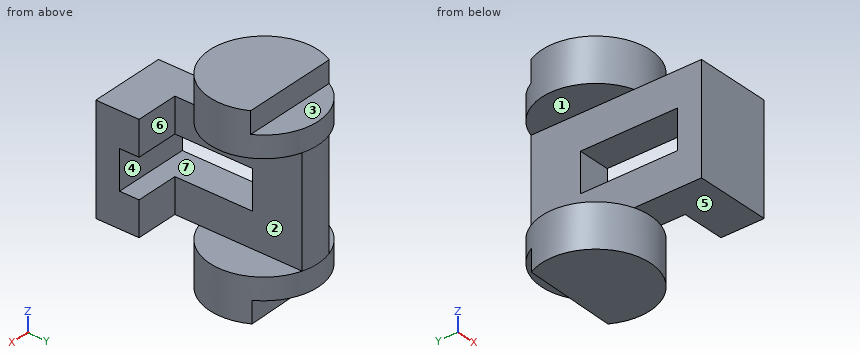
from build123d import *

# Parameters (mm, degrees)
BOSS_EXTRUDE1_DEPTH = 20
BOSS_EXTRUDE2_DEPTH = 50
SKETCH3_W           = 18
SKETCH3_H           = 45
CUT_EXTRUDE1_DEPTH  = 50
SKETCH4_R           = 25
BOSS_EXTRUDE3_DEPTH = 20
CUT_EXTRUDE2_START  = -10
CUT_EXTRUDE2_DEPTH  = 10
BOSS_EXTRUDE4_START = 50
BOSS_EXTRUDE4_DEPTH = 50
BOSS_EXTRUDE5_START = 20
SKETCH7_R           = 25
BOSS_EXTRUDE5_DEPTH = 20
CUT_EXTRUDE3_DEPTH  = 10


with BuildPart() as part:
    # Sketch1 → Boss-Extrude1 (new body)
    with BuildSketch(Plane(origin=(0, 0, 0), x_dir=(0, 0, -1), z_dir=(1, 0, 0))):
        Polygon((-22.633744856, 0), (-22.633744856, -20), (27.366255144, -20), (27.366255144, 0), (11.366255144, 0), (11.366255144, -9), (-6.633744856, -9), (-6.633744856, 0), align=None)
    extrude(amount=-BOSS_EXTRUDE1_DEPTH)

    # Sketch2 → Boss-Extrude2 (add)
    with BuildSketch(Plane.XY.offset(22.633744856)):
        Polygon((-20, 0), (-20, 54), (-35, 54), (-35, -20), (-20, -20), align=None)
    extrude(amount=-BOSS_EXTRUDE2_DEPTH)

    # Sketch3 → Cut-Extrude1 (cut)
    with BuildSketch(Plane(origin=(-20, 0, 0), x_dir=(0, 0, -1), z_dir=(1, 0, 0))):
        with Locations((2.366255144, 13.5)):
            Rectangle(SKETCH3_W, SKETCH3_H)
    extrude(amount=-CUT_EXTRUDE1_DEPTH, mode=Mode.SUBTRACT)

    # Sketch4 → Boss-Extrude3 (add)
    with BuildSketch(Plane.XY.offset(22.633744856)):
        with Locations(Location((-27.5, 35, 0), (0, 0, 252.542396876))):
            Circle(SKETCH4_R)
    extrude(amount=BOSS_EXTRUDE3_DEPTH)

    # Sketch5 → Cut-Extrude2 (cut)
    with BuildSketch(Plane.XY.offset(42.633744856).offset(CUT_EXTRUDE2_START)):
        with BuildLine():
            Line((-49.431712199, 47), (-5.568287801, 47))
            ThreePointArc((-5.568287801, 47), (-27.5, 60), (-49.431712199, 47))
        make_face()
    extrude(amount=CUT_EXTRUDE2_DEPTH, mode=Mode.SUBTRACT)

    # Sketch6 → Boss-Extrude4 (add)
    with BuildSketch(Plane(origin=(0, 0, 22.633744856), x_dir=(-1, 0, 0), z_dir=(0, 0, -1)).offset(BOSS_EXTRUDE4_START)):
        with BuildLine():
            Line((20, 54), (20, 58.848480035))
            ThreePointArc((20, 58.848480035), (27.5, 60), (35, 58.848480035))
            Line((35, 58.848480035), (35, 54))
            Line((35, 54), (20, 54))
        make_face()
    extrude(amount=-BOSS_EXTRUDE4_DEPTH)

    # Sketch7 → Boss-Extrude5 (add)
    with BuildSketch(Plane(origin=(0, 0, -27.366255144), x_dir=(-1, 0, 0), z_dir=(0, 0, -1)).offset(BOSS_EXTRUDE5_START)):
        with Locations((27.5, 35)):
            Circle(SKETCH7_R)
    extrude(amount=-BOSS_EXTRUDE5_DEPTH)

    # Sketch8 → Cut-Extrude3 (cut)
    with BuildSketch(Plane(origin=(0, 0, -47.366255144), x_dir=(-1, 0, 0), z_dir=(0, 0, -1))):
        with BuildLine():
            Line((5.820728213, 47.450268061), (49.674802071, 46.544615764))
            ThreePointArc((49.674802071, 46.544615764), (28.016177379, 59.99467065), (5.820728213, 47.450268061))
        make_face()
    extrude(amount=-CUT_EXTRUDE3_DEPTH, mode=Mode.SUBTRACT)


solid = part.part
Model file for the job. Use its own axes, mm. Face numbers are marked on the shaded views. A direction names the side the tool comes from. Give positions to 0.01 mm unless a question says otherwise; leave off trailing zeros. Loops run counter-clockwise (first coordinate to the right, second up) from the corner with the lowest first, then second, coordinate; pieces in that order, holes last. Notation, with made-up numbers: (44.25, 23) - (68.25, 23) arc R26 cw to (68.25, 40) - close; hole circle Ø2 at (72, 27.5). An arc over 180 degrees is marked (long way). Use one line per item in the form item = value.
(1) Drop flat-ended pins along their axis: P1, Ø5, axis at y = 49.5, z = -12, coming from the -X side; P2, Ø4, axis at x = -18.5, y = 52, coming from the +Z side; P3, Ø10, axis at y = 19.5, z = 13.5, coming from the +X side. Give the stop position or say it passes through.
Determined:
P1 = -35
P2 = 32.63
P3 = -20
(2) Cut at A-A (y = 20). Give the cut face in (x, z).
Determined:
outline = (-47.5, -47.37) - (-7.5, -47.37) - (-7.5, -27.37) - (-20, -27.37) - (-20, -11.37) - (-35, -11.37) - (-35, -27.37) - (-47.5, -27.37) - close; (-47.5, 22.63) - (-35, 22.63) - (-35, 6.63) - (-20, 6.63) - (-20, 22.63) - (-7.5, 22.63) - (-7.5, 42.63) - (-47.5, 42.63) - close
(3) Cut at D-D (y = 55). Give the cut face in (x, z), then the cut area to 3 significant figures.
Determined:
outline = (-42.5, -37.37) - (-12.5, -37.37) - (-12.5, -27.37) - (-20, -27.37) - (-20, 22.63) - (-12.5, 22.63) - (-12.5, 32.63) - (-42.5, 32.63) - (-42.5, 22.63) - (-35, 22.63) - (-35, -27.37) - (-42.5, -27.37) - close
area = 1,350 mm^2
(4) Pull direction Z, two halves, no side cores. Call the marked faces 5, 6 and 7: pulls with the +Z half, pulls with the -Z half, needs draft (parallel to the pull), parting line crosses it, or undercut.
Determined:
face_5 = pulls with the -Z half
face_6 = needs draft
face_7 = undercut
(5) Cut at B-B (x = -13.5). Give the cut face in (y, z), then the cut area to 3 significant figures.
Determined:
outline = (-20, -27.37) - (0, -27.37) - (0, -11.37) - (-9, -11.37) - (-9, 6.63) - (0, 6.63) - (0, 22.63) - (-20, 22.63) - close; (14.29, -47.37) - (47.29, -47.37) - (47.29, -37.37) - (55.71, -37.37) - (55.71, -27.37) - (14.29, -27.37) - close; (14.29, 22.63) - (55.71, 22.63) - (55.71, 32.63) - (47, 32.63) - (47, 42.63) - (14.29, 42.63) - close
area = 2,320 mm^2
(6) Drill centre lines: L1, parallel to Z at x = -38, y = 17.5; L2, parallel to Z at x = -23.5, y = 21; L3, parallel to X at y = 50, z = -4. Where is each one in solid material? Low to high.
Determined:
L1 = -47.37 to -27.37, 22.63 to 42.63
L2 = -47.37 to -11.37, 6.63 to 42.63
L3 = -35 to -20
(7) Cut at C-C (z = -2). Give the cut face in (x, y).
Determined:
outline = (-35, -20) - (0, -20) - (0, -9) - (-35, -9) - close; (-35, 36) - (-20, 36) - (-20, 58.85) arc R25 ccw to (-35, 58.85) - close
(8) 3-axis set-ups, long thin cutter, end or side, ignore diameter. For the marked faces 1, 2, 3 and 4: which of +Z, -Z, +X, -X, +Y, -Y reach the whole face in a straight line?
Determined:
face_1 = -X, +Y, -Y
face_2 = +X, +Y
face_3 = +Z, +X, -X, +Y
face_4 = +X, -X
